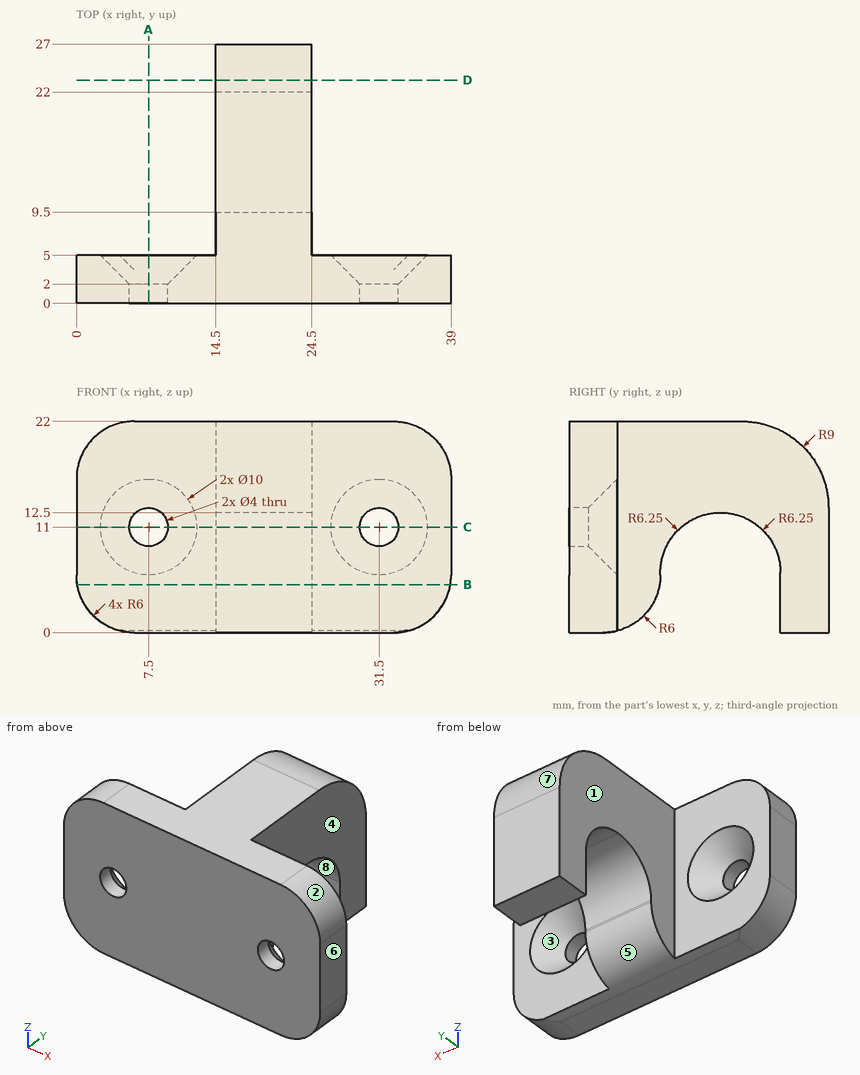
Job drawing, mm, ordinate dimensions from the low corner. One solid piece. A direction names the side the tool comes from. Coordinates: 2 decimals unless noted, no trailing zeros. Write each loop counter-clockwise with the first axis right and the second up, starting at its lowest first coordinate (ties: lowest second). Pieces come first, ordered by that corner, then holes. Notation, with made-up numbers: M 87,-4.5 L 100,-4.5 A11 ccw 100,13.5 Z; hole C 31.25,-4 d3. An arc over 180 degrees is marked long. Answer as a JSON object with one key per item and string values. Group by question number.
1) Mould opens along Y. For the marked faces 6, 7 and 8 say: +Y half, -Y half, draft (parallel to the pull), parting line (faces both ways), or undercut.
2) Saw through at B-B (z = 5). Write the cut outline in (x, y).
3) Tool access for the marked faces 1, 2, 3, 4 and 5: list every direction of +Z, -Z, +X, -X, +Y, -Y with a clear straight run to the whole face (end or side of a thin tool).
4) Saw through at A-A (x = 7.5). Write the cut outline in (y, z).
5) Wall check: line 1 (X direction, y = 1.4, z = 11); line 2 (X direction, y = 15.75, z = 19.5); line 3 (Y direction, x = 13.5, z = 10.75). Give the ranges that are in metal, low to high. Write a range as from..to.
6) Pin check, flat tips, straight feed: pin 1 Ø1 at (x, y) = (4, 4.5) entering from +Z; pin 2 Ø3.5 at (x, z) = (7.5, 11) entering from +Y; pin 3 Ø4.5 at (x, z) = (33.5, 6) entering from +Y; pin 4 Ø6 at (y, z) = (23.5, 12.5) entering from -X. Stop position of each tip, or through.
7) Saw through at C-C (z = 11). Write the cut outline in (x, y), plus the area to 3 significant figures.
8) Saw through at D-D (y = 23.25). Write the cut outline in (x, z), plus the area to 3 significant figures.
Values follow:
{
 "1": {"face 6": "draft", "face 7": "+Y half", "face 8": "undercut"},
 "2": {"outline": "M 0.08,0 L 38.92,0 L 38.92,5 L 24.5,5 L 24.5,9.42 L 14.5,9.42 L 14.5,5 L 0.08,5 Z; M 14.5,22 L 24.5,22 L 24.5,27 L 14.5,27 Z"},
 "3": {"face 1": "+Z, -Z, -X, +Y", "face 2": "+Z, +X, +Y, -Y", "face 3": "+Y", "face 4": "+Z, -Z, +X, +Y", "face 5": "-Z, +X, -X"},
 "4": {"outline": "M 0,0 L 3.5,0 A6 ccw 5,0.19 L 5,6 L 2,9 L 0,9 Z; M 0,13 L 2,13 L 5,16 L 5,22 L 0,22 Z"},
 "5": {"line 1": "x = 0..5.5, 9.5..29.5, 33.5..39", "line 2": "x = 14.5..24.5", "line 3": "y = 0..5"},
 "6": {"pin 1": "stops at z = 21.81", "pin 2": "passes through", "pin 3": "stops at y = 5", "pin 4": "stops at x = 14.5"},
 "7": {"outline": "M 0,0 L 5.5,0 L 5.5,2 L 2.5,5 L 0,5 Z; M 9.5,0 L 29.5,0 L 29.5,2 L 26.5,5 L 24.5,5 L 24.5,11.69 L 14.5,11.69 L 14.5,5 L 12.5,5 L 9.5,2 Z; M 14.5,19.81 L 24.5,19.81 L 24.5,27 L 14.5,27 Z; M 33.5,0 L 39,0 L 39,5 L 36.5,5 L 33.5,2 Z", "area": "276 mm2"},
 "8": {"outline": "M 14.5,0 L 24.5,0 L 24.5,20.31 L 14.5,20.31 Z", "area": "203 mm2"}
}
